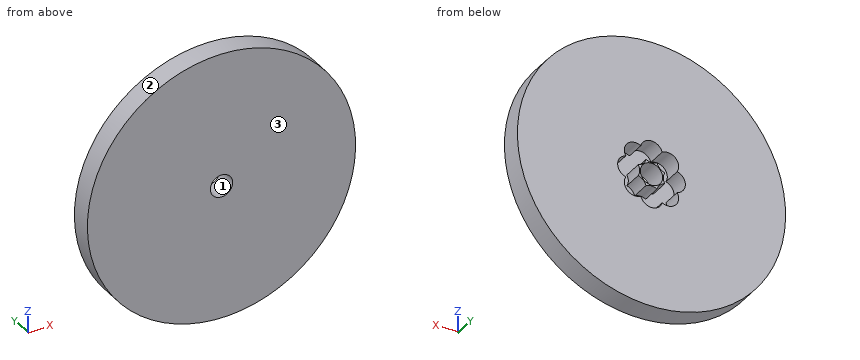
```python
from build123d import *

# Parameters (mm, degrees)
SKETCH1_R           = 60
BOSS_EXTRUDE1_DEPTH = 10
SKETCH2_R           = 5
CUT_EXTRUDE1_DEPTH  = 86.440037453
SKETCH3_R           = 4.931187375
CUT_EXTRUDE2_DEPTH  = 8.729106
CIRPATTERN1_START   = 1.270894058
CIRPATTERN1_DEPTH   = 8.729105942


# Read off the part's stored shape, not the designer's step: CirPattern1
with BuildPart() as part:
    # Sketch1 → Boss-Extrude1 (new body)
    with BuildSketch(Plane(origin=(0, 0, 0), x_dir=(1, 0, 0), z_dir=(0, 1, 0))):
        with Locations(Location((0, 0, 0), (0, 0, 270))):
            Circle(SKETCH1_R)
    extrude(amount=BOSS_EXTRUDE1_DEPTH)

    # Sketch2 → Cut-Extrude1 (cut, through all)
    with BuildSketch(Plane(origin=(0, 0, 0), x_dir=(1, 0, 0), z_dir=(0, 1, 0))):
        with Locations(Location((0, 0, 0), (0, 0, 270))):
            Circle(SKETCH2_R)
    extrude(amount=CUT_EXTRUDE1_DEPTH, mode=Mode.SUBTRACT)

    # Sketch3 → Cut-Extrude2 (cut)
    with BuildSketch(Plane(origin=(0, 10, 0), x_dir=(1, 0, 0), z_dir=(0, 1, 0))):
        with Locations(Location((-10.222069231, 0, 0), (0, 0, 270))):
            Circle(SKETCH3_R)
    extrude(amount=-CUT_EXTRUDE2_DEPTH, mode=Mode.SUBTRACT)

    # CirPattern1 outline → CirPattern1 (cut)
    with BuildSketch(Plane(origin=(0, 0, 0), x_dir=(1, 0, 0), z_dir=(0, 1, 0)).offset(CIRPATTERN1_START)):
        with BuildLine():
            ThreePointArc((2.465085219, -5.951242169), (0, -5.290881856), (-2.465085219, -5.951242169))
            ThreePointArc((-2.465085219, -5.951242169), (-3.741218439, -3.741218439), (-5.951242169, -2.465085219))
            ThreePointArc((-5.951242169, -2.465085219), (-8.334985521, -4.555823087), (-11.498921533, -4.763009251))
            ThreePointArc((-11.498921533, -4.763009251), (-10.714970503, -10.714970503), (-4.763009251, -11.498921533))
            ThreePointArc((-4.763009251, -11.498921533), (0, -15.153256606), (4.763009251, -11.498921533))
            ThreePointArc((4.763009251, -11.498921533), (10.714970503, -10.714970503), (11.498921533, -4.763009251))
            ThreePointArc((11.498921533, -4.763009251), (15.153256606, 0), (11.498921533, 4.763009251))
            ThreePointArc((11.498921533, 4.763009251), (10.714970503, 10.714970503), (4.763009251, 11.498921533))
            ThreePointArc((4.763009251, 11.498921533), (0, 15.153256606), (-4.763009251, 11.498921533))
            ThreePointArc((-4.763009251, 11.498921533), (-10.714970503, 10.714970503), (-11.498921533, 4.763009251))
            ThreePointArc((-11.498921533, 4.763009251), (-8.334985521, 4.555823087), (-5.951242169, 2.465085219))
            ThreePointArc((-5.951242169, 2.465085219), (-3.741218439, 3.741218439), (-2.465085219, 5.951242169))
            ThreePointArc((-2.465085219, 5.951242169), (0, 5.290881856), (2.465085219, 5.951242169))
            ThreePointArc((2.465085219, 5.951242169), (3.741218439, 3.741218439), (5.951242169, 2.465085219))
            ThreePointArc((5.951242169, 2.465085219), (5.290881856, 0), (5.951242169, -2.465085219))
            ThreePointArc((5.951242169, -2.465085219), (3.741218439, -3.741218439), (2.465085219, -5.951242169))
        make_face()
    extrude(amount=CIRPATTERN1_DEPTH, mode=Mode.SUBTRACT)


solid = part.part
```
Input: part model. Units: mm. Frame: model coordinates. Face numbers are marked on the shaded views. Coordinates: 2 decimals unless noted, no trailing zeros. Loops run counter-clockwise (first coordinate to the right, second up) from the corner with the lowest first, then second, coordinate; pieces in that order, holes last.
Q1. Section C-C, the plane z = 0. Return the cut outline in (x, y), and give its area (3 significant figures).
Results are:
outline: (-60, 0) - (-5, 0) - (-5, 10) - (-5.29, 10) - (-5.29, 1.27) - (-15.15, 1.27) - (-15.15, 10) - (-60, 10) - close; (5, 0) - (60, 0) - (60, 10) - (15.15, 10) - (15.15, 1.27) - (5.29, 1.27) - (5.29, 10) - (5, 10) - close
area: 928 mm2
Q2. Mould query, pull axis Z, two halves, no side actions, for the marked faces 1, 2 and 3. Classes: +Z half, -Z half, draft (parallel to the pull), parting line (faces both ways), or undercut.
Results are:
face 1: undercut
face 2: parting line
face 3: draft
Q3. Contact query for flat-ended pins moving along their axis: pin 1 (3 mm diameter, centred on y = 2, z = -26.5, fed in from +X); pin 2 (1 mm diameter, centred on x = 3.5, y = 3.5, fed in from -Z); pin 3 (6 mm diameter, centred on y = 2.5, z = 26, fed in from +X). Output: stop coordinate, or through.
Results are:
pin 1: stops at x = 54.54
pin 2: stops at z = -59.92
pin 3: stops at x = 55.42
Q4. Line query: line 1 along X through (y, z) = (3.75, 0); line 2 along Z through (x, y) = (-1, 6.75); line 3 along Z through (x, y) = (14, 2.75). Output: solid intervals per line, ascending.
Results are:
line 1: x = -60 to -15.15, -5.29 to -5, 5 to 5.29, 15.15 to 60
line 2: z = -59.99 to -15.05, -5.39 to -4.9, 4.9 to 5.39, 15.05 to 59.99
line 3: z = -58.34 to -3.17, 3.17 to 58.34
Q5. Section D-D, the plane x = -49.5. Return the cut outline in (y, z), and give its area (3 significant figures).
Results are:
outline: (0, -33.91) - (10, -33.91) - (10, 33.91) - (0, 33.91) - close
area: 678 mm2
Q6. Section B-B, the plane y = 7.75. Return the cut outline in (x, z).
Results are:
outline: circle Ø120 at (0, 0); (-5.95, -2.47) arc R4.93 cw to (-2.47, -5.95) arc R4.93 cw to (2.47, -5.95) arc R4.93 cw to (5.95, -2.47) arc R4.93 cw to (5.95, 2.47) arc R4.93 cw to (2.47, 5.95) arc R4.93 cw to (-2.47, 5.95) arc R4.93 cw to (-5.95, 2.47) arc R4.93 cw to start; hole (-11.5, -4.76) arc R4.93 ccw to (-4.76, -11.5) arc R4.93 ccw to (4.76, -11.5) arc R4.93 ccw to (11.5, -4.76) arc R4.93 ccw to (11.5, 4.76) arc R4.93 ccw to (4.76, 11.5) arc R4.93 ccw to (-4.76, 11.5) arc R4.93 ccw to (-11.5, 4.76) arc R4.93 ccw to start; hole circle Ø10 at (0, 0)
Q7. Section A-A, the plane x = 0. Return the cut outline in (y, z).
Results are:
outline: (0, -60) - (10, -60) - (10, -15.15) - (1.27, -15.15) - (1.27, -5.29) - (10, -5.29) - (10, -5) - (0, -5) - close; (0, 5) - (10, 5) - (10, 5.29) - (1.27, 5.29) - (1.27, 15.15) - (10, 15.15) - (10, 60) - (0, 60) - close
